from build123d import *

# Parameters (mm, degrees)
SALIENTE_EXTRUIR2_DEPTH = 2
CROQUIS4_R              = 1.5
SALIENTE_EXTRUIR3_DEPTH = 4
CROQUIS6_R              = 1.5
CORTAR_EXTRUIR1_DEPTH   = 44
CROQUIS7_R              = 2.7
CORTAR_EXTRUIR2_DEPTH   = 2
CORTAR_EXTRUIR3_DEPTH   = 2
CORTAR_EXTRUIR4_DEPTH   = 2
CROQUIS10_W             = 5
CROQUIS10_H             = 18
SALIENTE_EXTRUIR4_DEPTH = 2
SALIENTE_EXTRUIR5_DEPTH = 18
CROQUIS12_R             = 1.5
CORTAR_EXTRUIR5_DEPTH   = 5


with BuildPart() as part:
    # Croquis1 → Saliente-Extruir2 (new body)
    with BuildSketch(Plane(origin=(0, 0, 0), x_dir=(1, 0, 0), z_dir=(0, 1, 0))):
        with BuildLine():
            Line((3, 48), (18.129942315, 48))
            ThreePointArc((18.129942315, 48), (19.277992612, 47.771638598), (20.251262658, 47.121320344))
            Line((20.251262658, 47.121320344), (47.121320344, 20.251262658))
            ThreePointArc((47.121320344, 20.251262658), (47.771638598, 19.277992612), (48, 18.129942315))
            Line((48, 18.129942315), (48, 3))
            ThreePointArc((48, 3), (47.121320344, 0.878679656), (45, 0))
            Line((45, 0), (20.784609691, 0))
            ThreePointArc((20.784609691, 0), (18.820648679, 0.732213162), (17.815379735, 2.571428571))
            ThreePointArc((17.815379735, 2.571428571), (12.727922061, 12.727922061), (2.571428571, 17.815379735))
            ThreePointArc((2.571428571, 17.815379735), (0.732213162, 18.820648679), (0, 20.784609691))
            Line((0, 20.784609691), (0, 45))
            ThreePointArc((0, 45), (0.878679656, 47.121320344), (3, 48))
        make_face()
    extrude(amount=-SALIENTE_EXTRUIR2_DEPTH)

    # Croquis4 → Saliente-Extruir3 (add)
    with BuildSketch(Plane(origin=(0, 0, 0), x_dir=(1, 0, 0), z_dir=(0, 1, 0))):
        with BuildLine():
            Line((14.648353456, 0), (59.648353456, 0))
            ThreePointArc((59.648353456, 0), (62.020061701, -0.598295785), (63.824176728, -2.25))
            ThreePointArc((63.824176728, -2.25), (72.089608603, -2.37664761), (69.176765452, 5.359549678))
            ThreePointArc((69.176765452, 5.359549678), (29.192462946, 26.810912386), (4.755712821, 65.043760204))
            ThreePointArc((4.755712821, 65.043760204), (-0.781484452, 68.438550602), (-5, 63.5))
            Line((-5, 63.5), (-5, 54))
            ThreePointArc((-5, 54), (-6.464466094, 50.464466094), (-10, 49))
            Line((-10, 49), (-27, 49))
            Line((-27, 49), (-27, 15))
            Line((-27, 15), (-4.533601503, 15))
            ThreePointArc((-4.533601503, 15), (-2.464811146, 14.551934364), (-0.766802335, 13.288042583))
            ThreePointArc((-0.766802335, 13.288042583), (5.094474955, 7.035057245), (11.383817909, 1.212810057))
            ThreePointArc((11.383817909, 1.212810057), (12.907082327, 0.312999375), (14.648353456, 0))
        make_face()
        with Locations(Location((0, 63.5, 0), (0, 0, 270))):
            Circle(CROQUIS4_R, mode=Mode.SUBTRACT)
        with Locations(Location((68, 0.5, 0), (0, 0, 270))):
            Circle(CROQUIS4_R, mode=Mode.SUBTRACT)
    extrude(amount=SALIENTE_EXTRUIR3_DEPTH)

    # Croquis6 → Cortar-Extruir1 (cut)
    with BuildSketch(Plane.XZ.offset(2)):
        with Locations(Location((10.5, -32, 0), (0, 0, 270))):
            Circle(CROQUIS6_R)
        with Locations(Location((32, -10.5, 0), (0, 0, 270))):
            Circle(CROQUIS6_R)
    extrude(amount=-CORTAR_EXTRUIR1_DEPTH, mode=Mode.SUBTRACT)

    # Croquis7 → Cortar-Extruir2 (cut)
    with BuildSketch(Plane(origin=(0, 4, 0), x_dir=(1, 0, 0), z_dir=(0, 1, 0))):
        with Locations(Location((10.5, 32, 0), (0, 0, 270))):
            Circle(CROQUIS7_R)
        with Locations(Location((32, 10.5, 0), (0, 0, 270))):
            Circle(CROQUIS7_R)
    extrude(amount=-CORTAR_EXTRUIR2_DEPTH, mode=Mode.SUBTRACT)

    # Croquis8 → Cortar-Extruir3 (cut)
    with BuildSketch(Plane.XZ):
        Polygon((0, -60.324573519), (-2.75, -61.91228676), (-2.75, -65.08771324), (0, -66.675426481), (2.75, -65.08771324), (2.75, -61.91228676), align=None)
    extrude(amount=-CORTAR_EXTRUIR3_DEPTH, mode=Mode.SUBTRACT)

    # Croquis9 → Cortar-Extruir4 (cut)
    with BuildSketch(Plane.XZ):
        Polygon((64.824573519, -0.5), (66.41228676, -3.25), (69.58771324, -3.25), (71.175426481, -0.5), (69.58771324, 2.25), (66.41228676, 2.25), align=None)
    extrude(amount=-CORTAR_EXTRUIR4_DEPTH, mode=Mode.SUBTRACT)

    # Croquis10 → Saliente-Extruir4 (add)
    with BuildSketch(Plane(origin=(0, 4, 0), x_dir=(1, 0, 0), z_dir=(0, 1, 0))):
        with Locations((-3.5, 40)):
            Rectangle(CROQUIS10_W, CROQUIS10_H)
    extrude(amount=SALIENTE_EXTRUIR4_DEPTH)

    # Croquis11 → Saliente-Extruir5 (add)
    with BuildSketch(Plane.XY.offset(-31)):
        with BuildLine():
            Line((-6, 4), (-6, 13.5))
            Line((-6, 13.5), (-23, 13.5))
            Line((-23, 13.5), (-23, 16))
            Line((-23, 16), (-4, 16))
            ThreePointArc((-4, 16), (-1.878679656, 15.121320344), (-1, 13))
            Line((-1, 13), (-1, 4))
            Line((-1, 4), (-6, 4))
        make_face()
    extrude(amount=-SALIENTE_EXTRUIR5_DEPTH)

    # Croquis12 → Cortar-Extruir5 (cut)
    with BuildSketch(Plane(origin=(0, 16, 0), x_dir=(1, 0, 0), z_dir=(0, 1, 0))):
        with Locations(Location((-16, 40, 0), (0, 0, 270))):
            Circle(CROQUIS12_R)
    extrude(amount=-CORTAR_EXTRUIR5_DEPTH, mode=Mode.SUBTRACT)


solid = part.part
Verification items for the finished model (mm, model axes). A direction names the side the tool comes from. Round coordinates to 2 decimals unless told otherwise and drop trailing zeros. Loops run counter-clockwise (first coordinate to the right, second up) from the corner with the lowest first, then second, coordinate; pieces in that order, holes last. Notation, with made-up numbers: M -21,52 L -11,52 A25 cw -11,66 Z; hole C 56.25,17 d3. An arc over 180 degrees is marked long. Write each question's results on one line, items separated by ' | '.
1) Section check C-C on y = 14.75. Record the boundary of the cut face in (x, z).
Checks:
outline: M -23,-49 L -1.56,-49 L -1.56,-31 L -23,-31 Z; hole C -16,-40 d3
2) Access from +Z, -Z, +X, -X, +Y, -Y to the whole of each face (thin tool, end or side, straight path). Record for faces 1 (the flat face through (-2.75, 1, -63)), 2 (the flat face through (-1, 8, -40)), 3 (the flat face through (-7, 14, -49)), 4 (the flat face through (10, -1, -48)).
Checks:
face 1: -Y | face 2: +Z, -Z, +X, +Y | face 3: -Z, +X, -X, +Y | face 4: -Z, +X, -X, -Y
3) Gauge pin test, flat ends, axial feed: P1, Ø3, axis at x = 22, y = 0.5, coming from the -Z side; P2, Ø1.8, axis at x = 36.5, y = -0.5, coming from the +Z side; P3, Ø4.5, axis at x = -10, y = 2, coming from the +Z side. Record the tip position at first contact, or that the pin passes through.
Checks:
P1: stops at z = -46.79 | P2: stops at z = 0 | P3: stops at z = -15
4) Section check D-D on z = -40. Record the boundary of the cut face in (x, y), then the cut area to 3 significant figures.
Checks:
outline: M -27,0 L 0,0 L 0,-2 L 27.37,-2 L 27.37,0 L 17.5,0 L 17.5,4 L -1,4 L -1,13 A3 ccw -4,16 L -14.5,16 L -14.5,13.5 L -6,13.5 L -6,4 L -27,4 Z; M -23,13.5 L -17.5,13.5 L -17.5,16 L -23,16 Z | area: 326 mm2
5) Mould release check, pull along Z, two halves, no side actions. Record for faces 5 (the flat face through (68, 1, 2.25)), 6 (the cylindrical face through (18.843, -0.986, -0.713)), 7 (the flat face through (48, -1, -11)): released by +Z, released by -Z, zero draft, split by the parting line, or undercut.
Checks:
face 5: undercut | face 6: released by +Z | face 7: zero draft
6) Scan lines: L1, parallel to X at y = 14.65, z = -40; L2, parallel to Z at x = -11, y = 0.5; L3, parallel to Z at x = 0, y = 2.5. Record each from-to range of solid material in increasing order. Write a range as from..to.
Checks:
L1: x = -23..-17.5, -14.5..-1.49 | L2: z = -49..-15 | L3: z = -68.5..-65, -62..-12.42
7) Section check B-B on z = -10.5. Record the boundary of the cut face in (x, y), then the cut area to 3 significant figures.
Checks:
outline: M 1.74,0 L 14.62,0 L 14.62,-2 L 30.5,-2 L 30.5,2 L 29.3,2 L 29.3,4 L 1.74,4 Z; M 33.5,-2 L 48,-2 L 48,0 L 54.01,0 L 54.01,4 L 34.7,4 L 34.7,2 L 33.5,2 Z | area: 253 mm2
8) Section check A-A on x = -16. Record the boundary of the cut face in (y, z), then the cut area to 4 significant figures.
Checks:
outline: M 0,-49 L 4,-49 L 4,-15 L 0,-15 Z; M 13.5,-49 L 16,-49 L 16,-41.5 L 13.5,-41.5 Z; M 13.5,-38.5 L 16,-38.5 L 16,-31 L 13.5,-31 Z | area: 173.5 mm2
